```python
from build123d import *

# Parameters (mm, degrees)
SKETCH1_W            = 15
SKETCH1_H            = 82
BOSS_EXTRUDE1_DEPTH  = 10
SKETCH2_W            = 3
SKETCH2_H            = 15
CUT_EXTRUDE1_DEPTH   = 20
SKETCH3_R            = 1.55
SKETCH3_R_2          = 1.6
CUT_EXTRUDE2_DEPTH   = 10
FILLET1_START        = -17
FILLET1_DEPTH        = 17
FILLET1_START_2      = -15.76142132
FILLET1_2_DEPTH      = 15
FILLET3_R            = 1
SKETCH4_W            = 179.4
SKETCH4_H            = 5
BOSS_EXTRUDE3_DEPTH  = 10
FILLET3_OF_MIRROR3_R = 1
FILLET4_R            = 2
FILLET5_R            = 5
CUT_EXTRUDE3_REACH   = 193.882
SKETCH5_R            = 1.6


with BuildPart() as part:
    # Sketch1 → Boss-Extrude1 (new body)
    with BuildSketch(Plane.XY):
        with Locations((-8.26142132, -14.845177665)):
            Rectangle(SKETCH1_W, SKETCH1_H)
    boss_extrude1 = extrude(amount=BOSS_EXTRUDE1_DEPTH)

    # Sketch2 → Cut-Extrude1 (cut)
    with BuildSketch(Plane(origin=(-0.76142132, 0, 0), x_dir=(0, 0, -1), z_dir=(1, 0, 0))):
        with Locations((-1.5, 18.654822335)):
            Rectangle(SKETCH2_W, SKETCH2_H)
        with Locations((-8.5, 18.654822335)):
            Rectangle(SKETCH2_W, SKETCH2_H)
    cut_extrude1 = extrude(amount=-CUT_EXTRUDE1_DEPTH, mode=Mode.SUBTRACT)

    # Sketch3 → Cut-Extrude2 (cut, symmetric)
    with BuildSketch(Plane(origin=(0, 0, 3), x_dir=(-1, 0, 0), z_dir=(0, 0, -1))):
        with Locations(Location((4.26142132, 16.154822335, 0), (0, 0, 90))):
            Circle(SKETCH3_R)
        with Locations(Location((12.26142132, 16.154822335, 0), (0, 0, 90))):
            Circle(SKETCH3_R)
        with Locations(Location((8.26142132, -22.845177665, 0), (0, 0, 180))):
            Circle(SKETCH3_R_2)
    cut_extrude2 = extrude(amount=CUT_EXTRUDE2_DEPTH, both=True, mode=Mode.SUBTRACT)

    # Fillet1: read off the stored shape, not the designer's step
    # Fillet1 outline → Fillet1 (cut)
    with BuildSketch(Plane.YZ.offset(FILLET1_START)):
        with BuildLine():
            ThreePointArc((24.154822335, 7), (25.569035897, 6.414213562), (26.154822335, 5))
            Line((26.154822335, 5), (26.154822335, 7))
            Line((26.154822335, 7), (24.154822335, 7))
        make_face()
        with BuildLine():
            ThreePointArc((26.154822335, 5), (25.569035897, 3.585786438), (24.154822335, 3))
            Line((24.154822335, 3), (26.154822335, 3))
            Line((26.154822335, 3), (26.154822335, 5))
        make_face()
    fillet1 = extrude(amount=FILLET1_DEPTH, mode=Mode.SUBTRACT)

    # Fillet1 2 outline → Fillet1 2 (add)
    with BuildSketch(Plane.YZ.offset(FILLET1_START_2)):
        with BuildLine():
            Line((11.154822335, 7), (13.154822335, 7))
            ThreePointArc((13.154822335, 7), (11.740608773, 7.585786438), (11.154822335, 9))
            Line((11.154822335, 9), (11.154822335, 7))
        make_face()
        with BuildLine():
            ThreePointArc((11.154822335, 1), (11.740608773, 2.414213562), (13.154822335, 3))
            Line((13.154822335, 3), (11.154822335, 3))
            Line((11.154822335, 3), (11.154822335, 1))
        make_face()
    fillet1_2 = extrude(amount=FILLET1_2_DEPTH)

    # Fillet3
    fillet3_edges = [part.edges().sort_by_distance(p)[0] for p in [
        (-15.76142132, 11.154822335, 9.5),
        (-0.76142132, 11.154822335, 9.5),
        (-0.76142132, 11.154822335, 0.5),
        (-0.76142132, 18.654822335, 3),
        (-0.76142132, 18.654822335, 7),
        (-0.76142132, 25.569035897, 3.585786438),
        (-0.76142132, 25.569035897, 6.414213562),
        (-15.76142132, 18.654822335, 7),
        (-15.76142132, 18.654822335, 3),
        (-15.76142132, 11.154822335, 0.5),
        (-15.76142132, 25.569035897, 3.585786438),
        (-15.76142132, 25.569035897, 6.414213562),
        (-0.76142132, 11.740608773, 2.414213562),
        (-15.76142132, 11.740608773, 2.414213562),
        (-0.76142132, 11.740608773, 7.585786438),
        (-15.76142132, 11.740608773, 7.585786438),
    ]]
    fillet(fillet3_edges, radius=FILLET3_R)

    # Sketch4 → Boss-Extrude3 (add)
    with BuildSketch(Plane.XZ.offset(55.845177665)):
        with Locations((-90.46142132, 2.5)):
            Rectangle(SKETCH4_W, SKETCH4_H)
    extrude(amount=BOSS_EXTRUDE3_DEPTH)

    # Mirror3: Boss-Extrude1, Cut-Extrude1, Cut-Extrude2, Fillet1, Fillet1 2 across plane
    add(boss_extrude1.mirror(Plane.ZY.offset(90.46142132)))
    add(cut_extrude1.mirror(Plane.ZY.offset(90.46142132)), mode=Mode.SUBTRACT)
    add(cut_extrude2.mirror(Plane.ZY.offset(90.46142132)), mode=Mode.SUBTRACT)
    add(fillet1.mirror(Plane.ZY.offset(90.46142132)), mode=Mode.SUBTRACT)
    add(fillet1_2.mirror(Plane.ZY.offset(90.46142132)))

    # Fillet3 of Mirror3
    fillet3_of_mirror3_edges = [part.edges().sort_by_distance(p)[0] for p in [
        (-165.16142132, 11.154822335, 9.5),
        (-180.16142132, 11.154822335, 9.5),
        (-180.16142132, 11.154822335, 0.5),
        (-180.16142132, 18.654822335, 3),
        (-180.16142132, 18.654822335, 7),
        (-180.16142132, 25.569035897, 3.585786438),
        (-180.16142132, 25.569035897, 6.414213562),
        (-165.16142132, 18.654822335, 7),
        (-165.16142132, 18.654822335, 3),
        (-165.16142132, 11.154822335, 0.5),
        (-165.16142132, 25.569035897, 3.585786438),
        (-165.16142132, 25.569035897, 6.414213562),
        (-180.16142132, 11.740608773, 2.414213562),
        (-165.16142132, 11.740608773, 2.414213562),
        (-180.16142132, 11.740608773, 7.585786438),
        (-165.16142132, 11.740608773, 7.585786438),
    ]]
    fillet(fillet3_of_mirror3_edges, radius=FILLET3_OF_MIRROR3_R)

    # Fillet4
    fillet4_edges = [part.edges().sort_by_distance(p)[0] for p in [
        (-8.26142132, -55.845177665, 5),
        (-172.66142132, -55.845177665, 5),
    ]]
    fillet(fillet4_edges, radius=FILLET4_R)

    # Fillet5
    fillet5_edges = [part.edges().sort_by_distance(p)[0] for p in [
        (-15.76142132, -55.845177665, 2.5),
        (-180.16142132, -65.845177665, 2.5),
        (-0.76142132, -65.845177665, 2.5),
        (-165.16142132, -55.845177665, 2.5),
    ]]
    fillet(fillet5_edges, radius=FILLET5_R)

    # Sketch5 → Cut-Extrude3 (cut, up to next)
    with BuildSketch(Plane.XY.offset(5), mode=Mode.PRIVATE) as cut_extrude3_sk1:
        with Locations((-172.66142132, -60.845177665)):
            Circle(SKETCH5_R)
    cut_extrude3_tool1 = extrude(cut_extrude3_sk1.sketch, amount=-CUT_EXTRUDE3_REACH, mode=Mode.PRIVATE) & part.part
    # Sketch5 → Cut-Extrude3 (cut, up to next)
    with BuildSketch(Plane.XY.offset(5), mode=Mode.PRIVATE) as cut_extrude3_sk2:
        with Locations((-90.46142132, -60.845177665)):
            Circle(SKETCH5_R)
    cut_extrude3_tool2 = extrude(cut_extrude3_sk2.sketch, amount=-CUT_EXTRUDE3_REACH, mode=Mode.PRIVATE) & part.part
    # Sketch5 → Cut-Extrude3 (cut, up to next)
    with BuildSketch(Plane.XY.offset(5), mode=Mode.PRIVATE) as cut_extrude3_sk3:
        with Locations((-8.26142132, -60.845177665)):
            Circle(SKETCH5_R)
    cut_extrude3_tool3 = extrude(cut_extrude3_sk3.sketch, amount=-CUT_EXTRUDE3_REACH, mode=Mode.PRIVATE) & part.part
    add(cut_extrude3_tool1.solids().sort_by_distance((-172.661421, -60.845178, 5))[0], mode=Mode.SUBTRACT)
    add(cut_extrude3_tool2.solids().sort_by_distance((-90.461421, -60.845178, 5))[0], mode=Mode.SUBTRACT)
    add(cut_extrude3_tool3.solids().sort_by_distance((-8.261421, -60.845178, 5))[0], mode=Mode.SUBTRACT)


solid = part.part
```
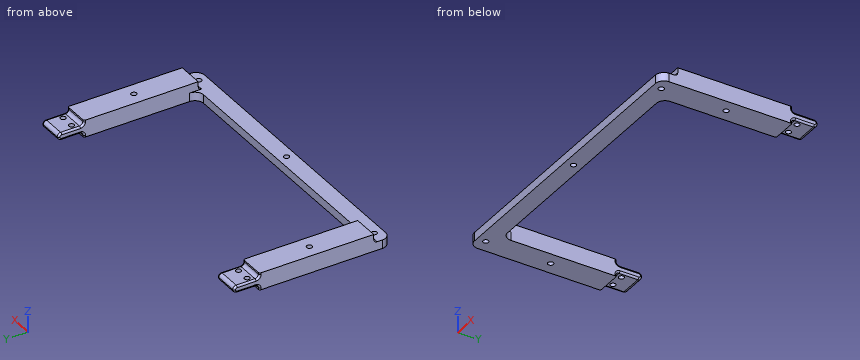
Build history of the part. All positions in model axes, mm. Round coordinates to 2 decimals unless told otherwise and drop trailing zeros. Write each loop counter-clockwise with the first axis right and the second up, starting at its lowest first coordinate (ties: lowest second). Pieces come first, ordered by that corner, then holes. Notation, with made-up numbers: (21, 59) -> (31, 59) arc R20 cw to (31, 83) -> close; hole circle Ø3 at (78.5, 5.25). An arc over 180 degrees is marked (long way). Put each result on its own line as item: value.
Item 1: Slice it at A-A, the plane y = -14.5. Give the cut face in (x, z), plus the area to 3 significant figures.
Here are the results:
outline: (-180.16, 0) -> (-165.16, 0) -> (-165.16, 10) -> (-180.16, 10) -> close; (-15.76, 0) -> (-0.76, 0) -> (-0.76, 10) -> (-15.76, 10) -> close
area: 300 mm^2
Item 2: Wall check: probe 1 along X at (y, z) = (-20, 7); probe 2 along Y at (x, z) = (-132, 3.5); probe 3 along Z at (x, y) = (-123, -61). Give the ranges that are in metal, low to high. Write a range as from..to.
Here are the results:
probe 1: x = -180.16..-165.16, -15.76..-0.76
probe 2: y = -65.85..-55.85
probe 3: z = 0..5
Item 3: Flat gauge pins, fed straight in: P1, Ø5, axis at x = -168.66, y = 16.15, coming from the -Z side; P2, Ø1.9, axis at x = -8.26, y = -22.85, coming from the +Z side; P3, Ø1.5, axis at x = -59.5, z = 2.5, coming from the +Y side; P4, Ø1.1, axis at x = -172, z = 0.5, coming from the +Y side. Where does each tip first touch, or does it go through?
Here are the results:
P1: stops at z = 3
P2: passes through
P3: stops at y = -55.85
P4: stops at y = 11.16
Item 4: Slice it at B-B, the plane x = -78. Give the cut face in (y, z).
Here are the results:
outline: (-65.85, 0) -> (-55.85, 0) -> (-55.85, 5) -> (-65.85, 5) -> close
